from build123d import *

# Parameters (mm, degrees)
F0_R     = 38.1
F1_DEPTH = 177.8
F4_D     = 36.11626
F4_DEPTH = 63.5
F4_TIP   = 10.8504191703
F5_SIZE2 = 12.7
F5_SIZE  = 25.4
F6_R     = 12.7
F7_W     = 25.4
F7_H     = 6.35
F8_DEPTH = 50.8


with BuildPart() as f1:
    # F0 (on Right) → F1 (new body)
    with BuildSketch(Plane.YZ):
        Circle(F0_R)
    extrude(amount=-F1_DEPTH)

    # F4
    with Locations(Plane.YZ):
        with Locations((0, 0)):
            Hole(F4_D / 2, depth=F4_DEPTH)
            with Locations((0, 0, -(F4_DEPTH + F4_TIP / 2))):  # 118° drill point
                Cone(0, F4_D / 2, F4_TIP, mode=Mode.SUBTRACT)

    # F5
    f5_edges = [f1.edges().sort_by_distance(p)[0] for p in [
        (-177.8, -38.1, 0),
    ]]
    f5_side = f1.faces().sort_by_distance((-88.9, -38.1, 0))[0]
    chamfer(f5_edges, length=F5_SIZE, length2=F5_SIZE2, reference=f5_side)

    # F6
    f6_edges = [f1.edges().sort_by_distance(p)[0] for p in [
        (-177.8, -25.4, 0),
        (-152.4, -38.1, 0),
    ]]
    fillet(f6_edges, radius=F6_R)

    # F7 (on Top) → F8 (cut, symmetric)
    with BuildSketch(Plane.XY):
        with Locations((-12.7, 34.925)):
            Rectangle(F7_W, F7_H)
        with Locations((-12.7, -34.925)):
            Rectangle(F7_W, F7_H)
    extrude(amount=F8_DEPTH, both=True, mode=Mode.SUBTRACT)


solid = f1.part
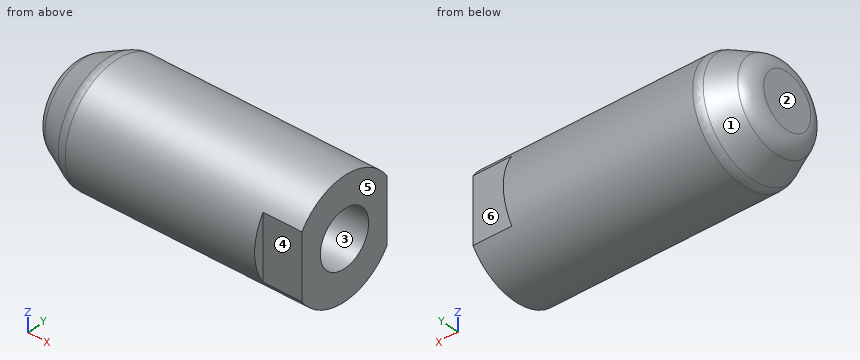
Geometry check sheet. Reference: the model listing, model coordinates, mm. Face numbers are marked on the shaded views. A direction names the side the tool comes from. Round coordinates to 2 decimals unless told otherwise and drop trailing zeros. Loops run counter-clockwise (first coordinate to the right, second up) from the corner with the lowest first, then second, coordinate; pieces in that order, holes last. Notation, with made-up numbers: (83, 69.5) -> (107, 69.5) arc R24 cw to (107, 86.5) -> close; hole circle Ø2 at (-40, 37). An arc over 180 degrees is marked (long way). Answer as a JSON object with one key per item and string values. Group by question number.
Item 1: Cross-section at B-B, the plane x = -157. Record the cut outline in (y, z), plus the area to 3 significant figures.
Item 2: Cross-section at C-C, the plane x = -84. Record the cut outline in (y, z), plus the area to 3 significant figures.
Item 3: Set-up check for the marked faces 4, 5 and 6: record each of +Z, -Z, +X, -X, +Y, -Y from which the full face is reachable in a straight line by a thin tool's end or side.
Item 4: Cross-section at A-A, the plane x = -23.5. Record the cut outline in (y, z), plus the area to 3 significant figures.
Item 5: Thickness scan on line 1 along Y through (x, z) = (-18, 0); line 2 along Z through (x, y) = (-38, 0). Record the ranges inside material, lowest first.
Item 6: Depth check by flat-ended pin: pin 1 Ø12 at (y, z) = (-26, -19) entering from -X; pin 2 Ø7.5 at (x, z) = (-8, -2) entering from +Y; pin 3 Ø1.9 at (y, z) = (35.5, -5) entering from +X. Enter the tip coordinate at first touch or a pass-through.
Item 7: Release check for a two-part mould opening along Z. For the marked faces 1, 2 and 3 record: pulls with the +Z half, pulls with the -Z half, needs draft (parallel to the pull), parting line crosses it, or undercut.
Determined:
{
 "1": {"outline": "circle Ø71.6 at (0, 0)", "area": "4,030 mm²"},
 "2": {"outline": "circle Ø76.2 at (0, 0)", "area": "4,560 mm²"},
 "3": {"face 4": "+Z, -Z, +X, -Y", "face 5": "+Z, -Z, +X, +Y, -Y", "face 6": "+Z, -Z, +X, +Y"},
 "4": {"outline": "(-31.75, -21.06) arc R38.1 ccw to (31.75, -21.06) -> (31.75, 21.06) arc R38.1 ccw to (-31.75, 21.06) -> close; hole circle Ø36.12 at (0, 0)", "area": "3,170 mm²"},
 "5": {"line 1": "y = -31.75 to -18.06, 18.06 to 31.75", "line 2": "z = -38.1 to -18.06, 18.06 to 38.1"},
 "6": {"pin 1": "stops at x = -174.4", "pin 2": "stops at y = 31.75", "pin 3": "stops at x = -25.4"},
 "7": {"face 1": "parting line crosses it", "face 2": "needs draft", "face 3": "undercut"}
}
